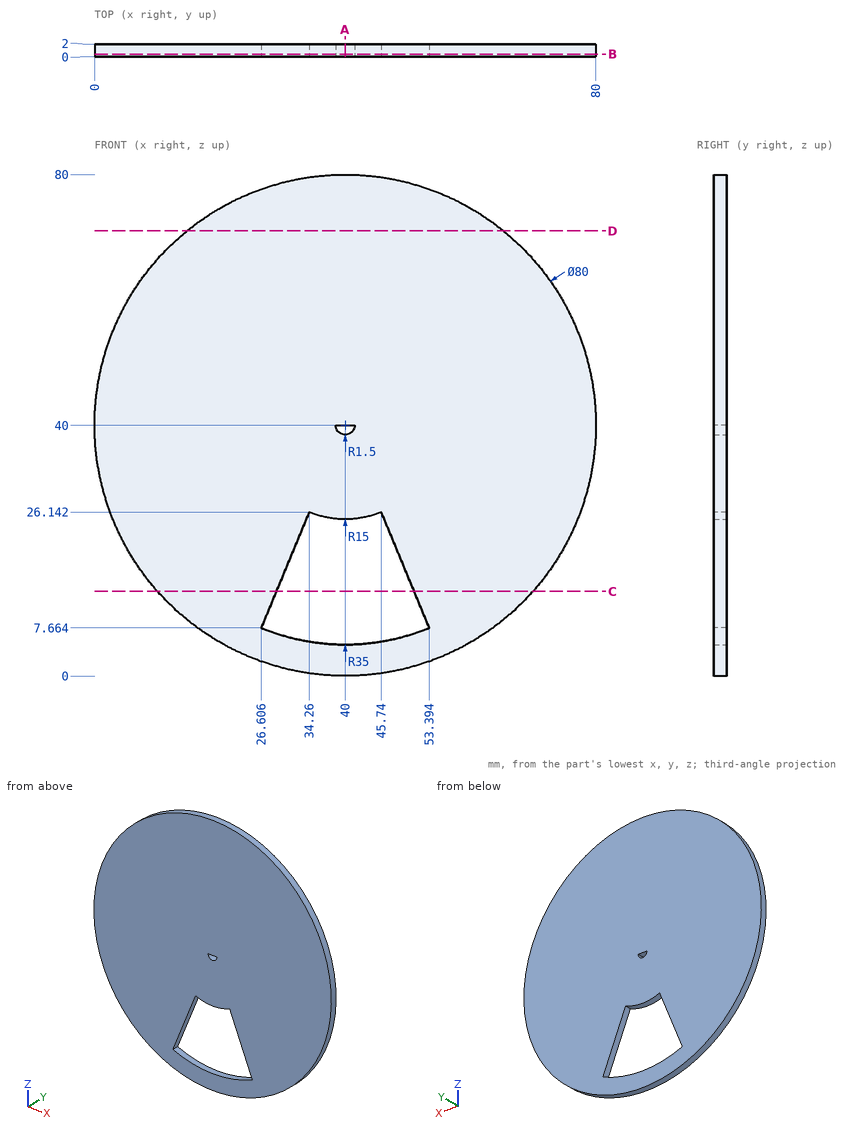
Input: dimensioned drawing with shaded views. Units: mm. Origin: part minimum x, y, z. Give positions to 0.01 mm unless a question says otherwise; leave off trailing zeros. Order: outer loops, then holes, each group sorted by start corner. A loop starts at its lowest first (then second) coordinate and runs counter-clockwise, first axis right, second up. Notation, with made-up numbers: (79.5, 69) -> (114.5, 69) arc R24 cw to (114.5, 96) -> close; hole circle Ø1 at (-1, 35). An arc over 180 degrees is marked (long way). Use a Markdown table: item, result.
1) Section query B-B, the plane y = 0.4. Return the cut outline in (x, z), then the cut area to 3 significant figures.
Answer list:
| item | result |
|---|---|
| outline | circle Ø80 at (40, 40); hole (26.61, 7.66) arc R35 ccw to (53.39, 7.66) -> (45.74, 26.14) arc R15 cw to (34.26, 26.14) -> close; hole (38.5, 40) arc R1.5 ccw to (41.5, 40) -> close |
| area | 4,630 mm² |
2) Section query D-D, the plane z = 71. Return the cut outline in (x, y), then the cut area to 3 significant figures.
Answer list:
| item | result |
|---|---|
| outline | (14.72, 0) -> (65.28, 0) -> (65.28, 2) -> (14.72, 2) -> close |
| area | 101 mm² |
3) Ray query, line 1 along X through (y, z) = (0.15, 15) (1 decimal); line 2 along X through (y, z) = (1.8, 41); line 3 along Z through (x, y) = (28.5, 1.05) (1 decimal). Return the intervals inside material, ascending. Write a range as [from, to].
Answer list:
| item | result |
|---|---|
| line 1 | [8.8, 29.6], [50.4, 71.2] |
| line 2 | [0.01, 79.99] |
| line 3 | [1.7, 6.9], [12.2, 78.3] |
4) Section query A-A, the plane x = 40. Return the cut outline in (y, z).
Answer list:
| item | result |
|---|---|
| outline | (0, 0) -> (2, 0) -> (2, 5) -> (0, 5) -> close; (0, 25) -> (2, 25) -> (2, 38.5) -> (0, 38.5) -> close; (0, 40) -> (2, 40) -> (2, 80) -> (0, 80) -> close |
5) Section query C-C, the plane z = 13.5. Return the cut outline in (x, y).
Answer list:
| item | result |
|---|---|
| outline | (10.04, 0) -> (29.02, 0) -> (29.02, 2) -> (10.04, 2) -> close; (50.98, 0) -> (69.96, 0) -> (69.96, 2) -> (50.98, 2) -> close |
6) Contact query for flat-ended pins moving along their axis: P1, Ø1, axis at x = 9.5, y = 0.5, coming from the -Z side; P2, Ø1, axis at x = 29.5, y = 0.5, coming from the -Z side. Output: stop coordinate, or through.
Answer list:
| item | result |
|---|---|
| P1 | z = 13.54 |
| P2 | z = 1.27 |
